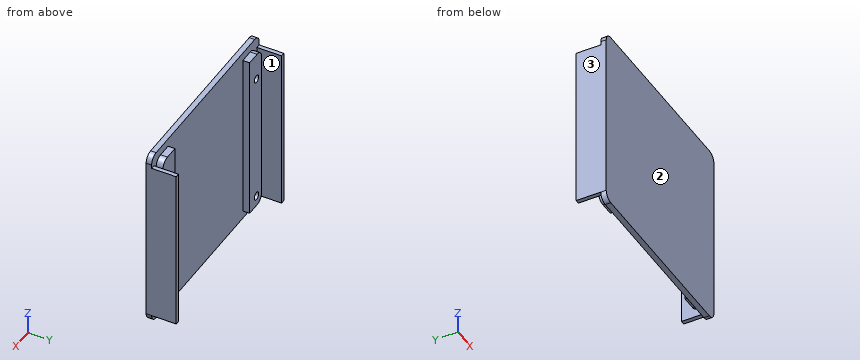
```python
from build123d import *

# Parameters (mm, degrees)
EXTRUDE_1_DEPTH = 2
SKETCH_3_W      = 1.5
SKETCH_3_H      = 60.659832998
EXTRUDE_2_DEPTH = 9
SKETCH_4_R      = 1.45
SKETCH_4_R_2    = 1.4
EXTRUDE_3_DEPTH = 2.5


with BuildPart() as part:
    # 草图2 → 凸台-拉伸1 (new body)
    with BuildSketch(Plane(origin=(0, 0, 0), x_dir=(1, 0, 0), z_dir=(0, 1, 0))):
        with BuildLine():
            Line((-33, 34), (33, 34))
            ThreePointArc((33, 34), (35.121320344, 33.121320344), (36, 31))
            Line((36, 31), (36, -31))
            ThreePointArc((36, -31), (35.121320344, -33.121320344), (33, -34))
            Line((33, -34), (-33, -34))
            ThreePointArc((-33, -34), (-35.121320344, -33.121320344), (-36, -31))
            Line((-36, -31), (-36, 31))
            ThreePointArc((-36, 31), (-35.121320344, 33.121320344), (-33, 34))
        make_face()
    extrude(amount=EXTRUDE_1_DEPTH)

    # 草图3 → 凸台-拉伸2 (add)
    with BuildSketch(Plane(origin=(0, 2, 0), x_dir=(1, 0, 0), z_dir=(0, 1, 0))):
        with Locations((-35.25, 0.670083501)):
            Rectangle(SKETCH_3_W, SKETCH_3_H)
        with Locations((35.25, 0.670083501)):
            Rectangle(SKETCH_3_W, SKETCH_3_H)
    extrude(amount=EXTRUDE_2_DEPTH)

    # 草图4 → 凸台-拉伸3 (add)
    # profile 1 of 2: a face of its own
    with BuildSketch(Plane(origin=(0, 2, 0), x_dir=(1, 0, 0), z_dir=(0, 1, 0))):
        with BuildLine():
            Line((-30, 31), (-25, 31))
            Line((-25, 31), (-25, -31))
            Line((-25, -31), (-30, -31))
            ThreePointArc((-30, -31), (-32.121320344, -30.121320344), (-33, -28))
            Line((-33, -28), (-33, 28))
            ThreePointArc((-33, 28), (-32.121320344, 30.121320344), (-30, 31))
        make_face()
        with Locations(Location((-29.6, 27.1, 0), (0, 0, 270))):
            Circle(SKETCH_4_R, mode=Mode.SUBTRACT)
        with Locations(Location((-29.6, -21.1, 0), (0, 0, 270))):
            Circle(SKETCH_4_R_2, mode=Mode.SUBTRACT)
    # profile 2 of 2: a face of its own
    with BuildSketch(Plane(origin=(0, 2, 0), x_dir=(1, 0, 0), z_dir=(0, 1, 0))):
        with BuildLine():
            Line((30, -31), (25, -31))
            Line((25, -31), (25, 31))
            Line((25, 31), (30, 31))
            ThreePointArc((30, 31), (32.121320344, 30.121320344), (33, 28))
            Line((33, 28), (33, -28))
            ThreePointArc((33, -28), (32.121320344, -30.121320344), (30, -31))
        make_face()
        with Locations(Location((29.6, 27.1, 0), (0, 0, 90))):
            Circle(SKETCH_4_R, mode=Mode.SUBTRACT)
        with Locations(Location((29.6, -21.1, 0), (0, 0, 90))):
            Circle(SKETCH_4_R_2, mode=Mode.SUBTRACT)
    extrude(amount=EXTRUDE_3_DEPTH)


solid = part.part
```
Verification items for the finished model (mm, model axes). Face numbers are marked on the shaded views. Give positions to 0.01 mm unless a question says otherwise; leave off trailing zeros. Loops run counter-clockwise (first coordinate to the right, second up) from the corner with the lowest first, then second, coordinate; pieces in that order, holes last. Notation, with made-up numbers: M 29,66.25 L 51,66.25 A13 ccw 51,72.25 Z; hole C 40.5,-8.5 d8. An arc over 180 degrees is marked long. One line per question, with ' | ' between items.
Item 1: Section check A-A, the plane y = 8.25. Record the cut outline in (x, z), plus the area to 3 significant figures.
Completed:
outline: M -36,-31 L -34.5,-31 L -34.5,29.66 L -36,29.66 Z; M 34.5,-31 L 36,-31 L 36,29.66 L 34.5,29.66 Z | area: 182 mm^2
Item 2: Section check D-D, the plane z = -27.1. Record the cut outline in (x, y).
Completed:
outline: M -36,0 L 36,0 L 36,11 L 34.5,11 L 34.5,2 L 33,2 L 33,4.5 L 31.05,4.5 L 31.05,2 L 28.15,2 L 28.15,4.5 L 25,4.5 L 25,2 L -25,2 L -25,4.5 L -28.15,4.5 L -28.15,2 L -31.05,2 L -31.05,4.5 L -33,4.5 L -33,2 L -34.5,2 L -34.5,11 L -36,11 Z
Item 3: Draft check along X on the marked faces 1, 2 and 3. Enter one of: +X half, -X half, draft (parallel to the pull), parting line (faces both ways), or undercut.
Completed:
face 1: undercut | face 2: draft | face 3: -X half
Item 4: Thickness scan on line 1 (Z direction, x = 29.6, y = 3.8); line 2 (X direction, y = 3.35, z = -27.1); line 3 (X direction, y = 4, z = -5). Record the ranges inside material, lowest first. Write a range as [from, to].
Completed:
line 1: z = [-31, -28.55], [-25.65, 19.7], [22.5, 31] | line 2: x = [-36, -34.5], [-33, -31.05], [-28.15, -25], [25, 28.15], [31.05, 33], [34.5, 36] | line 3: x = [-36, -34.5], [-33, -25], [25, 33], [34.5, 36]
Item 5: Section check B-B, the plane z = 8.5. Record the cut outline in (x, y), plus the area to 3 significant figures.
Completed:
outline: M -36,0 L 36,0 L 36,11 L 34.5,11 L 34.5,2 L 33,2 L 33,4.5 L 25,4.5 L 25,2 L -25,2 L -25,4.5 L -33,4.5 L -33,2 L -34.5,2 L -34.5,11 L -36,11 Z | area: 211 mm^2
Item 6: Depth check by flat-ended pin: P1, Ø0.9, axis at x = -29, z = -27.5, coming from the +Y side; P2, Ø5, axis at x = -18.5, y = 6.5, coming from the +Z side; P3, Ø2.5, axis at x = -31, z = 7, coming from the +Y side; P4, Ø1.2, axis at x = 28, y = 3, coming from the -Z side. Enter the tip coordinate at first touch or a pass-through.
Completed:
P1: stops at y = 2 | P2: passes through | P3: stops at y = 4.5 | P4: stops at z = -31
Item 7: Section check C-C, the plane x = -5.5. Record the cut outline in (y, z).
Completed:
outline: M 0,-34 L 2,-34 L 2,34 L 0,34 Z
